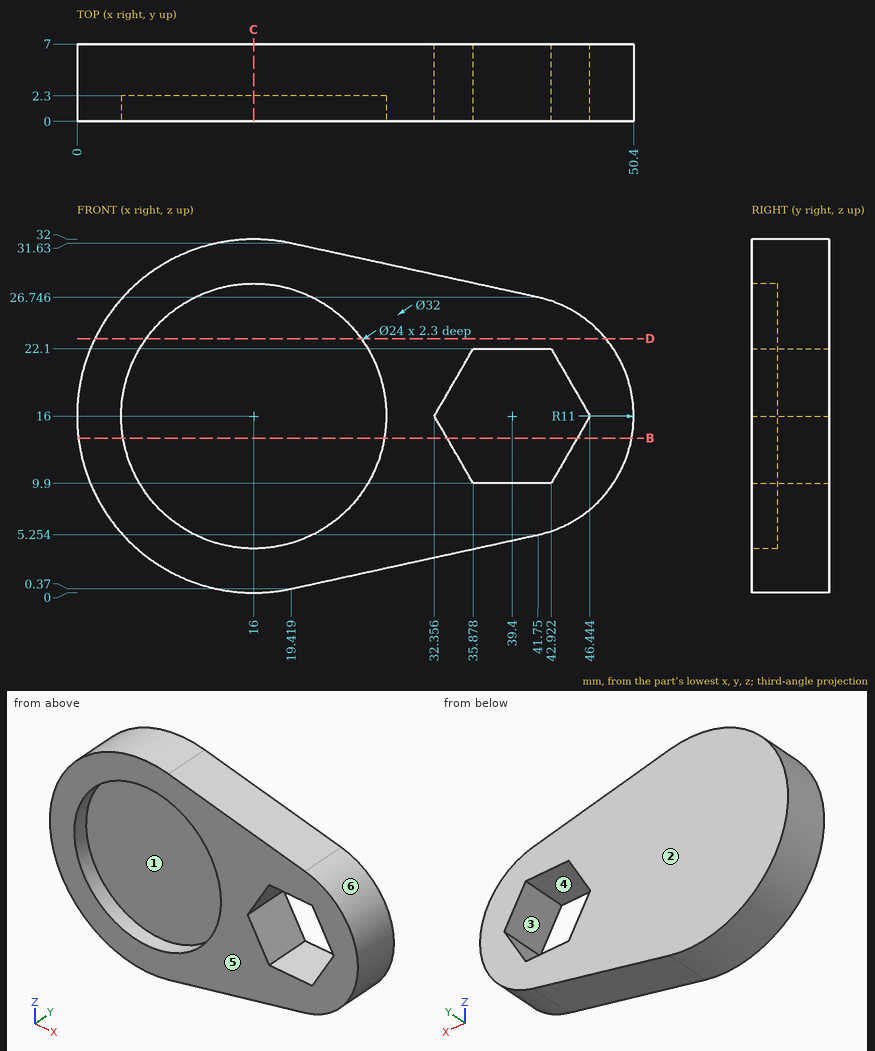
Input: dimensioned drawing with shaded views. Units: mm. Origin: part minimum x, y, z. A direction names the side the tool comes from. Coordinates: 2 decimals unless noted, no trailing zeros. Loops run counter-clockwise (first coordinate to the right, second up) from the corner with the lowest first, then second, coordinate; pieces in that order, holes last. Notation, with made-up numbers: (-33, 2) - (17, 2) arc R30 ccw to (17, 39) - close; hole circle Ø8 at (81.25, 35.5). An arc over 180 degrees is marked (long way). One line per question, with ' | ' between items. Start each with the question number.
(1) First-contact query: pin 1 (2 mm diameter, centred on x = 39.5, y = 5, fed in from -Z); pin 2 (14.5 mm diameter, centred on x = 16, z = 16, fed in from -Y); pin 3 (4 mm diameter, centred on x = 19, y = 1.5, fed in from +Z). Flat tips, straight axial feed; report the tip coordinate or a pass-through.
(2) Cut plane B-B on z = 14. Output: boundary loops of the cut face in (x, y) (1 decimal).
(3) Cut plane D-D on z = 23. Output: boundary loops of the cut face in (x, y) (1 decimal).
(4) Reachability of the marked faces 1, 2 and 3 from +Z, -Z, +X, -X, +Y, -Y: full face, straight path, thin tool, end or side. Return the list, or none.
(5) Draft query along X for the marked faces 4, 5 and 6. Return one class per face: +X half, -X half, draft (parallel to the pull), parting line (faces both ways), or undercut.
(6) Cut plane C-C on x = 16. Output: boundary loops of the cut face in (y, z).
(7) Ray query, L1, parallel to X at y = 0.7, z = 16 (1 decimal); L2, parallel to X at y = 0.75, z = 19 (1 decimal); L3, parallel to Y at x = 25.5, z = 12. Return the intervals inside material, ascending. Write a range as from..to.
Here are the results:
1) pin 1: z = 4.54 | pin 2: y = 2.3 | pin 3: z = 31.97
2) outline: (0.1, 0) - (4.2, 0) - (4.2, 2.3) - (27.8, 2.3) - (27.8, 0) - (33.5, 0) - (33.5, 7) - (0.1, 7) - close; (45.3, 0) - (50.2, 0) - (50.2, 7) - (45.3, 7) - close
3) outline: (1.6, 0) - (6.3, 0) - (6.3, 2.3) - (25.7, 2.3) - (25.7, 0) - (47.9, 0) - (47.9, 7) - (1.6, 7) - close
4) face 1: -Y | face 2: +Z, -Z, +X, -X, +Y | face 3: +Y, -Y
5) face 4: undercut | face 5: draft | face 6: +X half
6) outline: (0, 0) - (7, 0) - (7, 32) - (0, 32) - (0, 28) - (2.3, 28) - (2.3, 4) - (0, 4) - close
7) L1: 0..4, 28..32.4, 46.4..50.4 | L2: 0.3..4.4, 27.6..34.1, 44.7..50 | L3: 2.3..7
